Autodesk Inventor part; units mm, degrees
ref_plane "YZ Plane" through (0, 0, 0) normal (1, 0, 0) x (0, 1, 0)
ref_plane "XZ Plane" through (0, 0, 0) normal (0, 1, 0) x (-1, 0, 0)
ref_plane "XY Plane" through (0, 0, 0) normal (0, 0, 1) x (1, 0, 0)
sketch "Block1" plane through (0, 0, 0) normal (0, 0, 1) x (1, 0, 0)
  circle A0 centre (-3.2722, 18.9) radius 2.25
  circle A1 centre (-12.45, 7.7) radius 2.25
  circle A2 centre (-12.45, -4.3) radius 2.25
  line L0 (-6.45, -9) -> (-15.45, -9)
  line L1 (-6.45, -9) -> (-6.45, 12.4)
  line L2 (-6.45, 12.4) -> (2.9056, 12.4)
  line L3 (2.9056, 23.9) -> (-15.45, 23.9)
  line L4 (-15.45, -9) -> (-15.45, 23.9)
  line L5 (2.9056, 12.4) -> (2.9056, 23.9)
  line L6 (-6.45, 1.7) -> (-15.45, 1.7) construction
  point P0 (-7.0963, 8.6833)
  dimension "d131" = 6
  dimension "d132" = 6
sketch "Sketch1" plane through (0, 0, 0) normal (0, 0, 1) x (1, 0, 0)
  line L0 (-41.5, 50) -> (41.5, 50)
  line L1 (41.5, 50) -> (41.5, -50)
  line L2 (41.5, -50) -> (-41.5, -50)
  line L3 (-41.5, -50) -> (-41.5, 50)
  line L4 (31.5, 40) -> (-31.5, 40)
  line L5 (-31.5, 40) -> (-31.5, -40)
  line L6 (-31.5, -40) -> (31.5, -40)
  line L7 (31.5, -40) -> (31.5, 40)
  line L8 (-41.5, -45) -> (41.5, -45) construction
  line L9 (0, 71.7466) -> (0, -78.0681) construction
  line L10 (-60.2597, 0) -> (74.2823, 0) construction
  line L11 (-36.5, 50) -> (-36.5, -50) construction
  circle A0 centre (-36.5, -27) radius 2.25
  line L12 (-41.5, 45) -> (41.5, 45) construction
  circle A1 centre (-36.5, 45) radius 2.25
  circle A2 centre (-36.5, -45) radius 2.25
  circle A3 centre (-36.5, 27) radius 2.25
  circle A4 centre (-25, -45) radius 2.25
  circle A5 centre (25, -45) radius 2.25
  line L13 (30, 50) -> (30, -50) construction
  line L14 (-30, 50) -> (-30, -50) construction
  line L15 (-31, -38) -> (31, -38)
  line L16 (31, -38) -> (31, -52)
  line L17 (31, -52) -> (-31, -52)
  line L18 (-31, -52) -> (-31, -38)
  line L19 (-43.5, 33) -> (-29.5, 33)
  line L20 (-29.5, 33) -> (-29.5, -33)
  line L21 (-29.5, -33) -> (-43.5, -33)
  line L22 (-43.5, -33) -> (-43.5, 33)
  line L23 (-31.5, 40) -> (-24.5, 40)
  line L24 (-24.5, 40) -> (-24.5, 29)
  line L25 (-24.5, 29) -> (-31.5, 29)
  line L26 (-31.5, 29) -> (-31.5, 40)
  line L27 (-24.5, 29) -> (-29.5, 29)
  line L28 (-29.5, 29) -> (-29.5, 38)
  line L29 (-29.5, 38) -> (-24.5, 38)
  line L30 (-24.5, 38) -> (-24.5, 29)
  circle A6 centre (-27, 35.5) radius 1.5
  circle A7 centre (-27, 31.5) radius 1.5
  line L31 (22.2, -40) -> (-10.7, -40)
  point P0 (0, 0)
  point P1 (0, 50)
  point P2 (41.5, 0)
  point P3 (0, 45)
  point P4 (-27, 38)
  point P5 (-27, 29)
  dimension "d0" = 83
  dimension "d1" = 100
  dimension "d5" = 5
  dimension "d6" = 5
  dimension "d9" = 5
  dimension "d12" = 4.5
  dimension "d17" = 5
  dimension "d41" = 4.5
  dimension "d42" = 4.5
  dimension "d87" = 4.5
  dimension "d89" = 4.5
  dimension "d90" = 4.5
  dimension "d91" = 30
  dimension "d92" = 30
  dimension "d93" = 5
  dimension "d94" = 5
  dimension "d97" = 1
  dimension "d98" = 2
  dimension "d100" = 1
  dimension "d115" = 6
  dimension "d116" = 2
  dimension "d117" = 2
  dimension "d118" = 6
  dimension "d121" = 27
  dimension "d122" = 27
  dimension "d146" = 2
  dimension "d147" = 2
  dimension "d148" = 3
  dimension "d149" = 3
  dimension "d150" = 2.5
  dimension "d151" = 2.5
  dimension "d152" = 9
  dimension "d153" = 5
  dimension "d166" = 2
extrude "Extrusion1" add sketch "Sketch1" against normal blind 3 contours L0 L1 L2 L16 L6 L7 L4 L5 L19 L3 | L19 L5 L21 L3 | L21 L5 L6 L18 L2 L3 | L2 L18 L6 L16 | A0 | A1 | A2 | A3 | A4 | A5
extrude "Extrusion2" cut sketch "Sketch1" against normal blind 10 contours A0 | A1 | A2 | A3
mirror "Mirror1" about plane through (0, 0, 0) normal (1, 0, 0) of "Extrusion2"
extrude "Extrusion8" cut sketch "Sketch1" against normal blind 10 contours A4 | A5
extrude "Extrusion9" cut sketch "Sketch1" against normal blind 1 contours L16 L17 L18 L2 | L2 L18 L6 L16 | L6 L18 L15 L16
extrude "Extrusion14" add sketch "Sketch1" against normal blind 3 contours L19 L20 L25 L5 | L5 L4 L24 L29 L28 L19
extrude "Extrusion11" cut sketch "Sketch1" against normal blind 1 contours L19 L5 L21 L3 | L3 L21 L22 L19 | L19 L20 L25 L5 | L5 L25 L20 L21
mirror "Mirror4" about plane through (0, 0, 0) normal (0, 1, 0) of "Extrusion8", "Extrusion9"
mirror "Mirror5" about plane through (0, 0, 0) normal (1, 0, 0) of "Extrusion11"
extrude "Extrusion15" add sketch "Sketch1" against normal blind 3 contours L28 L29 L24 L25 L20
extrude "Extrusion16" add sketch "Sketch1" along normal blind 1.5 contours L28 L29 L24 L25 L20
mirror "Mirror6" about plane through (0, 0, 0) normal (1, 0, 0) of "Extrusion15", "Extrusion16", "Extrusion14"
mirror "Mirror7" about plane through (0, 0, 0) normal (0, 1, 0) of "Extrusion15", "Extrusion16", "Extrusion14", "Mirror6"
extrude "Extrusion18" cut sketch "Sketch1" against normal blind 1 contours L16 L17 L18 L2 | L2 L18 L6 L16 | L6 L18 L15 L16
extrude "Extrusion19" cut sketch "Sketch1" against normal blind 1 contours L19 L5 L21 L3 | L3 L21 L22 L19 | L19 L20 L25 L5 | L5 L25 L20 L21
mirror "Mirror8" about plane through (0, 0, 0) normal (1, 0, 0) of "Extrusion19"
equation "\"d12\" = screw"
equation "\"d41\" = screw"
equation "\"d42\" = screw"
equation "\"d87\" = screw"
equation "\"d89\" = screw"
equation "\"d90\" = screw"
equation "\"d37\" = mat"
properties part number "Side" material "PC/ABS Plastic"
The model under review builds one solid part; all positions refer to its coordinate system, in mm. A direction names the side the tool comes from. Give positions to 0.01 mm unless a question says otherwise; leave off trailing zeros. Order: outer loops, then holes, each group sorted by start corner. A loop starts at its lowest first (then second) coordinate and runs counter-clockwise, first axis right, second up. Notation, with made-up numbers: M -3,-17 L 36,-17 A14 cw 36,10 Z; hole C -35,47.25 d1. An arc over 180 degrees is marked long. Use one line per item in the form item = value. Start each with the question number.
Item 1: We need section C-C on y = 45. Give the boundary of the cut face in (x, z).
Item 2: The part is to be moulded in two halves that separate along X. For faces 3 (the flat face through (0, 40, -2)), 4 (the flat face through (-28, 38, 0)), 5 (the flat face through (41.5, 1, -2)), 6 (the flat face through (-27, -33.6, 1.5)), say which applies: pulls with the +X half, pulls with the -X half, needs draft (parallel to the pull), parting line crosses it, or undercut.
Item 3: We need section D-D on x = -36.5. Give the boundary of the cut face in (y, z), plus the area to 3 significant figures.
Item 4: To check wall thickness, follow line 1 along Y through (x, z) = (-27, -0.1); line 2 along X through (y, z) = (-35.5, -0.15); line 3 along Y through (x, z) = (36.5, -2.4). State the ranges of each line that lie inside material, in increasing order. Write a range as from..to.
Item 5: For faces 1 (the flat face through (-34, 4, -3)), 2 (the flat face through (24.5, 34, -1)), list the 3-axis set-ups (+Z, -Z, +X, -X, +Y, -Y) from which the entire face can be reached by the end or side of a thin tool; tool diameter is ignored.
Item 6: Insertion check: pin 1 Ø5 at (x, y) = (36.5, -27) entering from +Z; pin 2 Ø1.3 at (x, z) = (-28, 0) entering from -Y; pin 3 Ø7 at (x, y) = (-36.5, -45) entering from +Z. Each pin has a flat end and moves straight along its axis. Give the tip position at first contact, or say it passes through.
Item 7: We need section B-B on x = -3.5. Give the boundary of the cut face in (y, z).
Item 8: We need section A-A on y = -14.5. Give the boundary of the cut face in (x, z), plus the area to 3 significant figures.
Completed:
q1.outline = M -41.5,-3 L -38.75,-3 L -38.75,0 L -41.5,0 Z; M -34.25,-3 L -27.25,-3 L -27.25,-1 L -31,-1 L -31,0 L -34.25,0 Z; M -22.75,-3 L 22.75,-3 L 22.75,-1 L -22.75,-1 Z; M 27.25,-3 L 34.25,-3 L 34.25,0 L 31,0 L 31,-1 L 27.25,-1 Z; M 38.75,-3 L 41.5,-3 L 41.5,0 L 38.75,0 Z
q2.face_3 = undercut
q2.face_4 = undercut
q2.face_5 = pulls with the +X half
q2.face_6 = needs draft
q3.outline = M -50,-3 L -47.25,-3 L -47.25,0 L -50,0 Z; M -42.75,-3 L -29.25,-3 L -29.25,-1 L -33,-1 L -33,0 L -42.75,0 Z; M -24.75,-3 L 24.75,-3 L 24.75,-1 L -24.75,-1 Z; M 29.25,-3 L 42.75,-3 L 42.75,0 L 33,0 L 33,-1 L 29.25,-1 Z; M 47.25,-3 L 50,-3 L 50,0 L 47.25,0 Z
q3.area = 189 mm²
q4.line_1 = -38..-37, -34..-33, -30..-29, 29..30, 33..34, 37..38
q4.line_2 = -41.5..-28.5, -25.5..-24.5, 24.5..25.5, 28.5..41.5
q4.line_3 = -50..-47.25, -42.75..-29.25, -24.75..24.75, 29.25..42.75, 47.25..50
q5.face_1 = -Z, +X, -X, +Y, -Y
q5.face_2 = +Z, -Z
q6.pin_1 = -1
q6.pin_2 = -38
q6.pin_3 = 0
q7.outline = M -50,-3 L -40,-3 L -40,-1 L -50,-1 Z; M 40,-3 L 50,-3 L 50,-1 L 40,-1 Z
q8.outline = M -41.5,-3 L -31.5,-3 L -31.5,-1 L -41.5,-1 Z; M 31.5,-3 L 41.5,-3 L 41.5,-1 L 31.5,-1 Z
q8.area = 40.0 mm²
